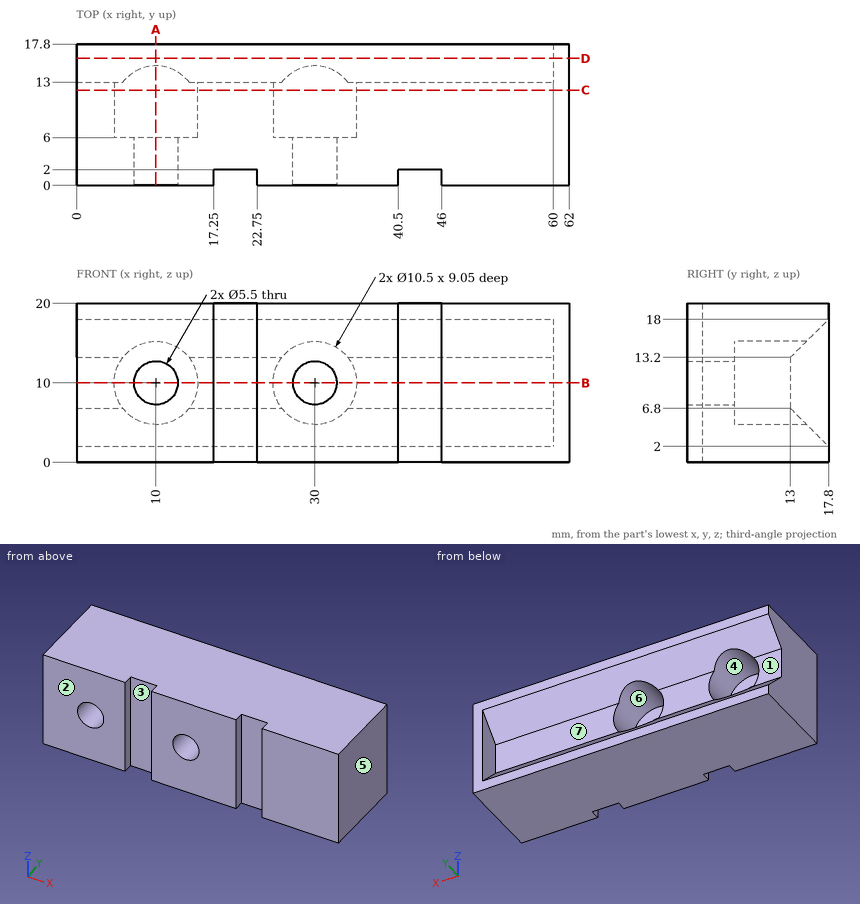
Job drawing, mm, ordinate dimensions from the low corner. One solid piece. A direction names the side the tool comes from. Give positions to 0.01 mm unless a question says otherwise; leave off trailing zeros. Loops run counter-clockwise (first coordinate to the right, second up) from the corner with the lowest first, then second, coordinate; pieces in that order, holes last. Notation, with made-up numbers: M 42.25,3.25 L 96.25,3.25 A30 ccw 96.25,30.25 Z; hole C -27.75,76 d9. An arc over 180 degrees is marked long. Use one line per item in the form item = value.
Item 1: Slice it at B-B on z = 10. Give the number of separate pieces and of enclosed holes in the cut face, and give its area (3 significant figures).
Filled in:
separate_pieces = 3
enclosed_holes = 0
area = 581 mm^2
Item 2: Slice it at A-A on x = 10. List the corners of the cut face in (y, z).
Filled in:
outline = M 0,0 L 17.8,0 L 17.8,2 L 15.05,4.75 L 6,4.75 L 6,7.25 L 0,7.25 Z; M 0,12.75 L 6,12.75 L 6,15.25 L 15.05,15.25 L 17.8,18 L 17.8,20 L 0,20 Z
Item 3: Slice it at C-C on y = 12. List the corners of the cut face in (x, z), and give its area (3 significant figures).
Filled in:
outline = M 0,0 L 62,0 L 62,20 L 0,20 Z; hole C 10,10 d10.5; hole C 30,10 d10.5
area = 1,070 mm^2
Item 4: Slice it at D-D on y = 16. List the corners of the cut face in (x, z), and give its area (3 significant figures).
Filled in:
outline = M 0,0 L 62,0 L 62,20 L 0,20 L 0,16.2 L 60,16.2 L 60,3.8 L 0,3.8 Z
area = 496 mm^2
Item 5: Two-plate mould, pull along X, no slides. Class the marked faces 5, 6 and 7: released by +X, released by -X, zero draft, split by the parting line, or undercut.
Filled in:
face_5 = released by +X
face_6 = undercut
face_7 = zero draft
Item 6: Drill centre lines: L1, parallel to X at y = 4.75, z = 10; L2, parallel to X at y = 9.25, z = 10; L3, parallel to Z at x = 30, y = 4.7. Where is each one in solid material? Low to high.
Filled in:
L1 = 0 to 7.25, 12.75 to 27.25, 32.75 to 62
L2 = 0 to 4.75, 15.25 to 24.75, 35.25 to 62
L3 = 0 to 7.25, 12.75 to 20
Item 7: Flat gauge pins, fed straight in: pin 1 Ø3.5 at (x, z) = (10, 10) entering from +Y; pin 2 Ø1.9 at (x, z) = (22.5, 10) entering from +Y; pin 3 Ø4.5 at (x, z) = (2.5, 11.5) entering from +Y; pin 4 Ø3 at (x, z) = (7.5, 12) entering from +Y. Where does each tip first touch, or does it go through?
Filled in:
pin_1 = through
pin_2 = 13
pin_3 = 13.55
pin_4 = 6
Item 8: Which spindle directions (+Z, -Z, +X, -X, +Y, -Y) get a long thin tool onto all of the face, cutting with end or side? Do the marked faces 1, 2, 3 and 4. Say none if no direction does.
Filled in:
face_1 = -X, +Y
face_2 = +Z, -Z, +X, -X, -Y
face_3 = +Z, -Z, -Y
face_4 = +Y
